Geometry check sheet. Reference: the model listing, model coordinates, mm. Face numbers are marked on the shaded views. Give positions to 0.01 mm unless a question says otherwise; leave off trailing zeros. Loops run counter-clockwise (first coordinate to the right, second up) from the corner with the lowest first, then second, coordinate; pieces in that order, holes last. Notation, with made-up numbers: (-10, -9) -> (40, -9) arc R25 cw to (40, 9) -> close; hole circle Ø8 at (35, 48.25). An arc over 180 degrees is marked (long way). Write each question's results on one line, items separated by ' | '. Start each with the question number.
1) Depth check by flat-ended pin: pin 1 (13 mm diameter, centred on x = 0, y = 130, fed in from +Z); pin 2 (6 mm diameter, centred on x = -14.5, z = -3, fed in from +Y). Enter the tip coordinate at first touch or a pass-through.
2) Sectioned sample at B-B on x = 0. Record the cut outline in (y, z).
3) Sectioned sample at A-A on y = 130. Record the cut outline in (x, z).
4) Scan lines: line 1 (Y direction, x = 0, z = 0.75); line 2 (Y direction, x = -1.5, z = -3); line 3 (Y direction, x = 17.5, z = 0.75). Record each from-to range of solid material in increasing order. Write a range as from..to.
5) Sectioned sample at D-D on x = -7. Record the cut outline in (y, z).
6) Draft check along Y on the marked faces 1, 2, 3 and 4. Enter one of: pulls with the +Y half, pulls with the -Y half, needs draft (parallel to the pull), parting line crosses it, or undercut.
7) Sectioned sample at C-C on z = -3.5. Record the cut outline in (x, y), then the cut area to 3 significant figures.
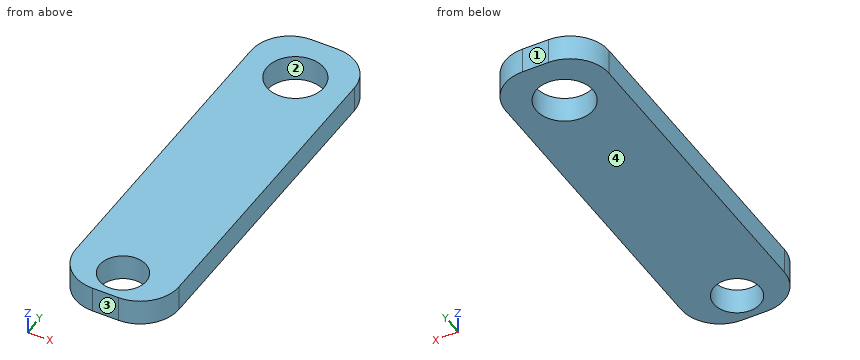
```python
from build123d import *

# Parameters (mm, degrees)
SKIZZE1_W                       = 40
SKIZZE1_H                       = 10
AUFSATZ_LINEAR_AUSTRAGEN1_DEPTH = 150
SKIZZE2_R                       = 11
SCHNITT_LINEAR_AUSTRAGEN1_DEPTH = 152.657508881
SKIZZE3_R                       = 9
SCHNITT_LINEAR_AUSTRAGEN5_DEPTH = 152.657508881
VERRUNDUNG1_R                   = 15


with BuildPart() as part:
    # Skizze1 → Aufsatz-Linear austragen1 (new body)
    with BuildSketch(Plane(origin=(0, 0, 0), x_dir=(1, 0, 0), z_dir=(0, 1, 0))):
        Rectangle(SKIZZE1_W, SKIZZE1_H)
    extrude(amount=AUFSATZ_LINEAR_AUSTRAGEN1_DEPTH)

    # Skizze2 → Schnitt-Linear austragen1 (cut, through all)
    with BuildSketch(Plane.XY.offset(5)):
        with Locations((0, 130)):
            Circle(SKIZZE2_R)
    extrude(amount=-SCHNITT_LINEAR_AUSTRAGEN1_DEPTH, mode=Mode.SUBTRACT)

    # Skizze3 → Schnitt-Linear austragen5 (cut, through all)
    with BuildSketch(Plane.XY.offset(5)):
        with Locations((0, 12)):
            Circle(SKIZZE3_R)
    extrude(amount=-SCHNITT_LINEAR_AUSTRAGEN5_DEPTH, mode=Mode.SUBTRACT)

    # Verrundung1
    verrundung1_edges = [part.edges().sort_by_distance(p)[0] for p in [
        (-20, 150, 0),
        (20, 150, 0),
        (-20, 0, 0),
        (20, 0, 0),
    ]]
    fillet(verrundung1_edges, radius=VERRUNDUNG1_R)


solid = part.part
```
Result:
1) pin 1: through | pin 2: y = 148.52
2) outline: (0, -5) -> (3, -5) -> (3, 5) -> (0, 5) -> close; (21, -5) -> (119, -5) -> (119, 5) -> (21, 5) -> close; (141, -5) -> (150, -5) -> (150, 5) -> (141, 5) -> close
3) outline: (-20, -5) -> (-11, -5) -> (-11, 5) -> (-20, 5) -> close; (11, -5) -> (20, -5) -> (20, 5) -> (11, 5) -> close
4) line 1: 0..3, 21..119, 141..150 | line 2: 0..3.13, 20.87..119.1, 140.9..150 | line 3: 6.71..143.29
5) outline: (0.13, -5) -> (6.34, -5) -> (6.34, 5) -> (0.13, 5) -> close; (17.66, -5) -> (121.51, -5) -> (121.51, 5) -> (17.66, 5) -> close; (138.49, -5) -> (149.87, -5) -> (149.87, 5) -> (138.49, 5) -> close
6) face 1: pulls with the +Y half | face 2: undercut | face 3: pulls with the -Y half | face 4: needs draft
7) outline: (-20, 15) arc R15 ccw to (-5, 0) -> (5, 0) arc R15 ccw to (20, 15) -> (20, 135) arc R15 ccw to (5, 150) -> (-5, 150) arc R15 ccw to (-20, 135) -> close; hole circle Ø22 at (0, 130); hole circle Ø18 at (0, 12) | area: 5,170 mm^2
